Check sheet for the modelled part. Datum: model origin and axes. Units: mm. A direction names the side the tool comes from. Give positions to 0.01 mm unless a question says otherwise; leave off trailing zeros. Write each loop counter-clockwise with the first axis right and the second up, starting at its lowest first coordinate (ties: lowest second). Pieces come first, ordered by that corner, then holes. Notation, with made-up numbers: (-1, 23) -> (37, 23) arc R32 cw to (37, 57) -> close; hole circle Ø8 at (23, 45). An arc over 180 degrees is marked (long way). Use a Markdown table: item, result. Add a question column.
1. Cross-section at D-D (y = -50.5). Enter the section's corners in (x, z).
2. Release check for a two-part mould opening along X. For faces 5 (the flat face through (12, 0, -7)), 6 (the flat face through (27.5, -39, -25)), 7 (the conical face through (12.3, 15.466, -13.51)), 8 (the flat face through (0, -39, -30)) record: released by +X, released by -X, zero draft, split by the parting line, or undercut.
3. Cross-section at A-A (y = -96.5). Enter the section's corners in (x, z).
4. Cross-section at B-B (x = 0). Enter the section's corners in (y, z), then the cut area to 3 significant figures.
5. Gauge pin test, flat ends, axial feed: P1, Ø5, axis at x = -22.5, y = -28.5, coming from the +Z side; P2, Ø1.5, axis at y = -30, z = -19, coming from the -X side; P3, Ø2.5, axis at x = -9.5, z = -21.5, coming from the -Y side. Record the tip position at first contact, or that the pin passes through.
6. Set-up check for faces 1 (the flat face through (22, -39, -20)), 2 (the flat face through (-27.5, -39, -25)), 3 (the cylindrical face through (12.368, -33.013, -22.395)), 4 (the flat face through (12, 0, -23)): record each of +Z, -Z, +X, -X, +Y, -Y from which the full face is reachable in a straight line by a thin tool's end or side.
7. Cross-section at C-C (y = 9). Enter the section's corners in (x, z).
8. Scan lines: probe 1 along Y at (x, z) = (-12.5, -18.5); probe 2 along X at (y, z) = (23.75, -23); probe 3 along Z at (x, y) = (12.5, 3.75). Record each from-to range of solid material in increasing order. Write a range as [from, to].
Autodesk Inventor part; units mm, degrees
ref_plane "YZ Plane" through (0, 0, 0) normal (1, 0, 0) x (0, 1, 0)
ref_plane "XZ Plane" through (0, 0, 0) normal (0, 1, 0) x (-1, 0, 0)
ref_plane "XY Plane" through (0, 0, 0) normal (0, 0, 1) x (1, 0, 0)
sketch "Sketch1" plane through (0, 0, 0) normal (0, 1, 0) x (-1, 0, 0)
  line L0 (17.5, 0) -> (-17.5, 0)
  line L1 (27.5, -30) -> (-27.5, -30)
  line L2 (27.5, -30) -> (27.5, -20)
  line L3 (27.5, -20) -> (17.5, -20)
  line L4 (-27.5, -30) -> (-27.5, -20)
  line L5 (-27.5, -20) -> (-17.5, -20)
  line L6 (17.5, -20) -> (17.5, 0)
  line L7 (-17.5, -20) -> (-17.5, 0)
  circle A0 centre (12.5, -23) radius 3
  circle A1 centre (-12.5, -23) radius 3
  circle A2 centre (-12.5, -7) radius 3
  circle A3 centre (12.5, -7) radius 3
  point P0 (0, 0)
  dimension "d2" = 35
  dimension "d8" = 55
  dimension "d9" = 10
  dimension "d10" = 10
  dimension "d11" = 6
  dimension "d12" = 6
  dimension "d13" = 6
  dimension "d14" = 6
  dimension "d17" = 7
  dimension "d18" = 16
extrude "Extrusion1" add sketch "Sketch1" along normal blind 30
sketch "Sketch4" plane through (0, 0, 0) normal (0, -1, 0) x (1, 0, 0)
  line L0 (27.5, -20) -> (27.5, -30)
  line L1 (27.5, -30) -> (-27.5, -30)
  line L2 (27.5, -30) -> (-27.5, -30)
  line L3 (-27.5, -30) -> (-27.5, -20)
  line L4 (-27.5, -30) -> (-27.5, -20)
  line L5 (-27.5, -20) -> (-17.5, -20)
  line L6 (-27.5, -20) -> (-17.5, -20)
  line L7 (-17.5, -20) -> (-17.5, 0)
  line L8 (-17.5, -20) -> (-17.5, 0)
  line L9 (-17.5, 0) -> (17.5, 0)
  line L10 (-17.5, 0) -> (17.5, 0)
  line L11 (17.5, 0) -> (17.5, -20)
  line L12 (17.5, 0) -> (17.5, -20)
  line L13 (17.5, -20) -> (27.5, -20)
  line L14 (27.5, -20) -> (27.5, -30)
  point P0 (0, 0)
extrude "Extrusion3" add sketch "Sketch4" along normal blind 70
sketch "Sketch5" plane through (0, -70, 0) normal (0, -1, 0) x (1, 0, 0)
  line L0 (27.5, -30) -> (-27.5, -30)
  line L1 (27.5, -30) -> (-27.5, -30)
  line L2 (-27.5, -30) -> (-27.5, -20)
  line L3 (-27.5, -30) -> (-27.5, -20)
  line L4 (-27.5, -20) -> (-17.5, -20)
  line L5 (-27.5, -20) -> (-17.5, -20)
  line L6 (-17.5, -20) -> (-17.5, 0)
  line L7 (-17.5, -20) -> (-17.5, 0)
  line L8 (-17.5, 0) -> (17.5, 0)
  line L9 (17.5, 0) -> (17.5, -20)
  line L10 (17.5, 0) -> (17.5, -20)
  line L11 (17.5, -20) -> (27.5, -20)
  line L12 (17.5, -20) -> (27.5, -20)
  line L13 (27.5, -20) -> (27.5, -30)
  line L14 (27.5, -20) -> (27.5, -30)
  circle A0 centre (0, -8) radius 4
  circle A1 centre (10.5, -23) radius 4
  circle A2 centre (-10.5, -23) radius 4
  point P0 (0, 0)
  dimension "d25" = 8
  dimension "d26" = 8
  dimension "d27" = 8
  dimension "d28" = 10.5
  dimension "d29" = 10.5
  dimension "d30" = 8
  dimension "d31" = 15
extrude "Extrusion4" add sketch "Sketch5" along normal blind 40
sketch "Sketch6" plane through (27.5, 30, -30) normal (0, 0, -1) x (-1, 0, 0)
  circle A0 centre (40, -105.0156) radius 3
  circle A1 centre (15, -105.0156) radius 3
  circle A2 centre (15, -60.0156) radius 3
  line L0 (55, -140) -> (0, -140)
  line L1 (27.5, 4.7422) -> (27.5, -229.8437)
  line L2 (55, -140) -> (55, 0)
  circle A3 centre (40, -60.0156) radius 3
  circle A4 centre (15, -15.0156) radius 3
  circle A5 centre (40, -15.0156) radius 3
  point P0 (27.5, -30)
  dimension "d35" = 6
  dimension "d38" = 6
  dimension "d39" = 6
  dimension "d42" = 45
  dimension "d43" = 27.5
  dimension "d44" = 12.5
  dimension "d53" = 6
  dimension "d54" = 6
  dimension "d55" = 6
  dimension "d56" = 45
  dimension "d57" = 45
hole "Hole1" at (-12.5, -75.0156, -30) at (12.5, -75.0156, -30) at (-12.5, -30.0156, -30) at (12.5, -30.0156, -30) at (12.5, 14.9844, -30) at (-12.5, 14.9844, -30) direction (0, 0, 1) diameter 6 depth 15 tip angle 118
properties part number "Fuhrung" material "Steel"
Worked answers:
| question | item | result |
|---|---|---|
| 1 | outline | (-27.5, -30) -> (27.5, -30) -> (27.5, -20) -> (17.5, -20) -> (17.5, 0) -> (-17.5, 0) -> (-17.5, -20) -> (-27.5, -20) -> close |
| 2 | face 5 | undercut |
| 2 | face 6 | released by +X |
| 2 | face 7 | undercut |
| 2 | face 8 | zero draft |
| 3 | outline | (-27.5, -30) -> (27.5, -30) -> (27.5, -20) -> (17.5, -20) -> (17.5, 0) -> (-17.5, 0) -> (-17.5, -20) -> (-27.5, -20) -> close; hole circle Ø8 at (-10.5, -23); hole circle Ø8 at (0, -8); hole circle Ø8 at (10.5, -23) |
| 4 | outline | (-110, -30) -> (30, -30) -> (30, 0) -> (-110, 0) -> (-110, -4) -> (-70, -4) -> (-70, -12) -> (-110, -12) -> close |
| 4 | area | 3,880 mm² |
| 5 | P1 | stops at z = -20 |
| 5 | P2 | stops at x = -17.5 |
| 5 | P3 | stops at y = -70 |
| 6 | face 1 | +Z, +X, +Y, -Y |
| 6 | face 2 | +Z, -Z, -X, +Y, -Y |
| 6 | face 3 | -Z |
| 6 | face 4 | +Y |
| 7 | outline | (-27.5, -30) -> (27.5, -30) -> (27.5, -20) -> (17.5, -20) -> (17.5, 0) -> (-17.5, 0) -> (-17.5, -20) -> (-27.5, -20) -> close; hole circle Ø6 at (-12.5, -23); hole circle Ø6 at (-12.5, -7); hole circle Ø6 at (12.5, -23); hole circle Ø6 at (12.5, -7) |
| 8 | probe 1 | y = [-110, -78.02], [-72.02, -33.02], [-27.02, 11.98], [17.98, 30] |
| 8 | probe 2 | x = [-27.5, -15.5], [-9.5, 9.5], [15.5, 27.5] |
| 8 | probe 3 | z = [-30, -26], [-20, -10], [-4, 0] |
